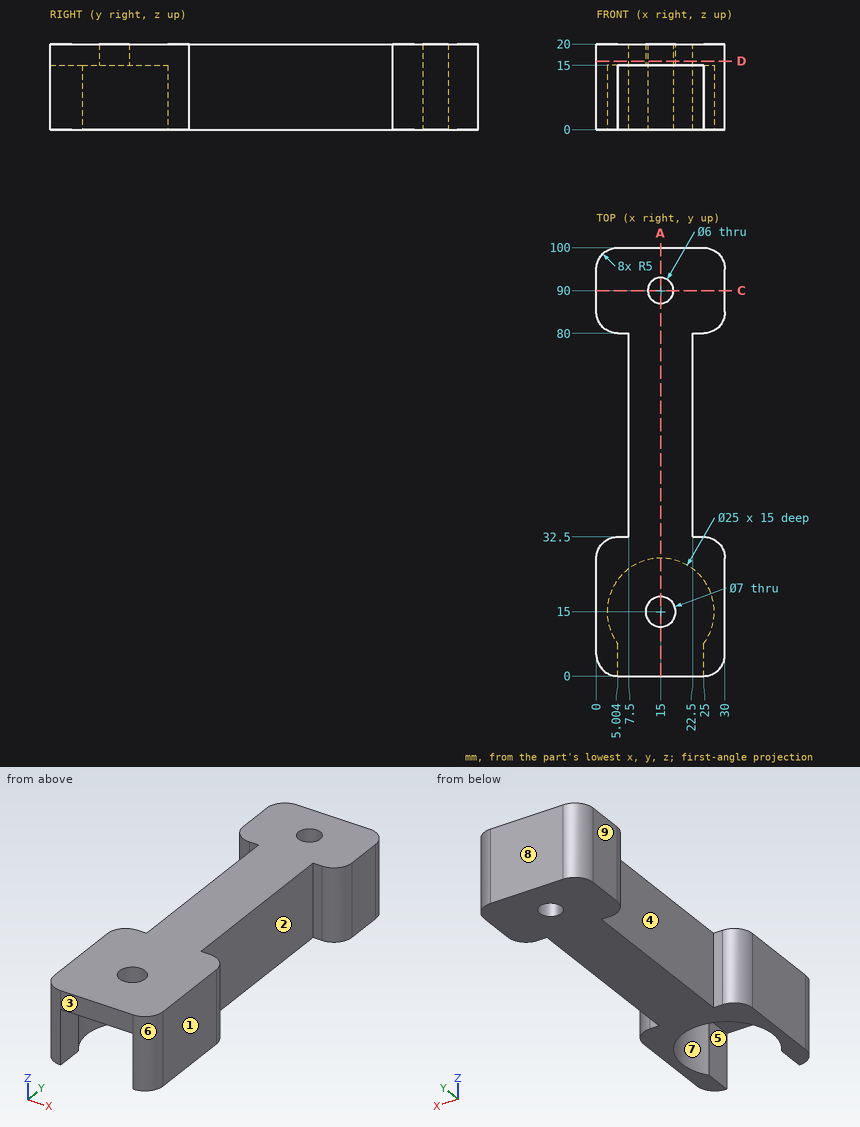
Check sheet for the drawn part. Datum: minimum x, y, z corner. Units: mm. A direction names the side the tool comes from. Give positions to 0.01 mm unless a question says otherwise; leave off trailing zeros. Order: outer loops, then holes, each group sorted by start corner. A loop starts at its lowest first (then second) coordinate and runs counter-clockwise, first axis right, second up.
1. Access from +Z, -Z, +X, -X, +Y, -Y to the whole of each face (thin tool, end or side, straight path). Record for the marked faces 1, 2, 3, 4 and 5.
Completed:
face 1: +Z, -Z, +X, +Y, -Y
face 2: +Z, -Z, +X
face 3: +Z, -Z, +X, -X, -Y
face 4: +Z, -Z, -X
face 5: -Z, -Y
2. Sectioned sample at C-C (y = 90). Record the boundary of the cut face in (x, z).
Completed:
outline: (0, 0) - (12, 0) - (12, 20) - (0, 20) - close; (18, 0) - (30, 0) - (30, 20) - (18, 20) - close
3. Sectioned sample at A-A (x = 15). Record the boundary of the cut face in (y, z), then the cut area to 3 significant figures.
Completed:
outline: (0, 15) - (11.5, 15) - (11.5, 20) - (0, 20) - close; (18.5, 15) - (27.5, 15) - (27.5, 0) - (87, 0) - (87, 20) - (18.5, 20) - close; (93, 0) - (100, 0) - (100, 20) - (93, 20) - close
area: 1,430 mm2
4. Depth check by flat-ended pin: pin 1 (12 mm diameter, centred on y = 37.5, z = 5.5, fed in from +X); pin 2 (6 mm diameter, centred on y = 3, z = 5, fed in from -X); pin 3 (6 mm diameter, centred on y = 62.5, z = 11, fed in from +X); pin 4 (5 mm diameter, centred on y = 58, z = 3, fed in from -X). Enter the tip coordinate at first touch or a pass-through.
Completed:
pin 1: stops at x = 28
pin 2: stops at x = 0
pin 3: stops at x = 22.5
pin 4: stops at x = 7.5
5. Draft check along X on the marked faces 6, 7, 8 and 9. Enter one of: pulls with the +X half, pulls with the -X half, needs draft (parallel to the pull), parting line crosses it, or undercut.
Completed:
face 6: pulls with the +X half
face 7: undercut
face 8: needs draft
face 9: pulls with the -X half
6. Sectioned sample at D-D (z = 16). Record the boundary of the cut face in (x, y).
Completed:
outline: (0, 5) arc R5 ccw to (5, 0) - (25, 0) arc R5 ccw to (30, 5) - (30, 27.5) arc R5 ccw to (25, 32.5) - (22.5, 32.5) - (22.5, 80) - (25, 80) arc R5 ccw to (30, 85) - (30, 95) arc R5 ccw to (25, 100) - (5, 100) arc R5 ccw to (0, 95) - (0, 85) arc R5 ccw to (5, 80) - (7.5, 80) - (7.5, 32.5) - (5, 32.5) arc R5 ccw to (0, 27.5) - close; hole circle Ø7 at (15, 15); hole circle Ø6 at (15, 90)
7. Scan lines: line 1 (Y direction, x = 15, z = 18.95); line 2 (Y direction, x = 15, z = 5.75); line 3 (X direction, y = 15, z = 11). Record each from-to range of solid material in increasing order.
Completed:
line 1: y = 0 to 11.5, 18.5 to 87, 93 to 100
line 2: y = 27.5 to 87, 93 to 100
line 3: x = 0 to 2.5, 27.5 to 30
